from build123d import *

# Parameters (mm, degrees)
SKETCH1_W               = 50
SKETCH1_H               = 100
BOSS_EXTRUDE1_DEPTH     = 10
CUT_EXTRUDE1_DEPTH      = 72.414284285
CUT_EXTRUDE1_DEPTH_BACK = 72.414284285
SKETCH2_R               = 3.104362215
SKETCH2_R_2             = 3.085158395
SKETCH2_R_3             = 3.1
SKETCH2_R_4             = 3.004524649
CUT_EXTRUDE2_DEPTH      = 72.414284285
CUT_EXTRUDE2_DEPTH_BACK = 72.414284285
SKETCH4_R               = 1.557412487
SKETCH4_R_2             = 1.55


with BuildPart() as part:
    # Sketch1 → Boss-Extrude1 (new body)
    with BuildSketch(Plane(origin=(0, 0, 0), x_dir=(1, 0, 0), z_dir=(0, 1, 0))):
        with Locations((-25, 0)):
            Rectangle(SKETCH1_W, SKETCH1_H)
    extrude(amount=BOSS_EXTRUDE1_DEPTH)

    # Sketch2 → Cut-Extrude1 (cut, two sides: drawn at the far end of the back side and taken through both)
    with BuildSketch(Plane(origin=(0, 10, 0), x_dir=(1, 0, 0), z_dir=(0, 1, 0)).offset(-CUT_EXTRUDE1_DEPTH_BACK)):
        with Locations(Location((-32.847308623, -43.305370298, 0), (0, 0, 270))):
            Circle(SKETCH2_R)
        with Locations(Location((-43.698787397, -32.453891525, 0), (0, 0, 270))):
            Circle(SKETCH2_R_2)
        with Locations(Location((-21.99582985, -32.453891525, 0), (0, 0, 270))):
            Circle(SKETCH2_R_3)
        with Locations(Location((-32.847308623, -21.602412752, 0), (0, 0, 270))):
            Circle(SKETCH2_R)
        with Locations(Location((-32.847308623, -32.453891525, 0), (0, 0, 270))):
            Circle(SKETCH2_R_4)
        with Locations(Location((-32.847308623, 32.453891525, 0), (0, 0, 270))):
            Circle(SKETCH2_R_4)
        with Locations(Location((-32.847308623, 21.602412752, 0), (0, 0, 270))):
            Circle(SKETCH2_R)
        with Locations(Location((-21.99582985, 32.453891525, 0), (0, 0, 270))):
            Circle(SKETCH2_R_3)
        with Locations(Location((-43.698787397, 32.453891525, 0), (0, 0, 270))):
            Circle(SKETCH2_R_2)
        with Locations(Location((-32.847308623, 43.305370298, 0), (0, 0, 270))):
            Circle(SKETCH2_R)
    extrude(amount=CUT_EXTRUDE1_DEPTH + CUT_EXTRUDE1_DEPTH_BACK, mode=Mode.SUBTRACT)

    # Sketch4 → Cut-Extrude2 (cut, two sides: drawn at the far end of the back side and taken through both)
    with BuildSketch(Plane(origin=(0, 10, 0), x_dir=(1, 0, 0), z_dir=(0, 1, 0)).offset(-CUT_EXTRUDE2_DEPTH_BACK)):
        with Locations(Location((-41.474384237, 10.515205344, 0), (0, 0, 270))):
            Circle(SKETCH4_R)
        with Locations(Location((-41.474384237, -10.343457517, 0), (0, 0, 270))):
            Circle(SKETCH4_R_2)
        with Locations(Location((-31.474384237, -10.343457517, 0), (0, 0, 270))):
            Circle(SKETCH4_R_2)
        with Locations(Location((-31.474384237, 10.515205344, 0), (0, 0, 270))):
            Circle(SKETCH4_R)
        with Locations(Location((-21.474384237, 10.515205344, 0), (0, 0, 270))):
            Circle(SKETCH4_R_2)
        with Locations(Location((-21.474384237, -10.343457517, 0), (0, 0, 270))):
            Circle(SKETCH4_R_2)
        with Locations(Location((-11.474384237, -10.343457517, 0), (0, 0, 270))):
            Circle(SKETCH4_R_2)
        with Locations((-1.474384237, -10.343457517)):
            Circle(SKETCH4_R_2)
        with Locations(Location((-11.474384237, 10.515205344, 0), (0, 0, 270))):
            Circle(SKETCH4_R)
        with Locations((-1.474384237, 10.515205344)):
            Circle(SKETCH4_R)
    extrude(amount=CUT_EXTRUDE2_DEPTH + CUT_EXTRUDE2_DEPTH_BACK, mode=Mode.SUBTRACT)


solid = part.part
Verification items for the finished model (mm, model axes). Coordinates: 2 decimals unless noted, no trailing zeros. Loops run counter-clockwise (first coordinate to the right, second up) from the corner with the lowest first, then second, coordinate; pieces in that order, holes last. Notation, with made-up numbers: (82.25, 53.25) -> (110.25, 53.25) arc R33 ccw to (110.25, 84.25) -> close; hole circle Ø5 at (37.5, -13). An arc over 180 degrees is marked (long way). Answer as CSV lines item,"result".
1) Cross-section at C-C, the plane y = 6. Count the separate pieces of the cut face and the enclosed holes in it, then the cut area to 3 significant figures.
Found:
separate pieces,"1"
enclosed holes,"18"
area,"4,630 mm2"
2) Release check for a two-part mould opening along Z. For faces 1 (the flat face through (-25, 0, -1)), 2 (the flat face through (-25, 5, -50)), 3 (the cylindrical face through (-35.78, 4.93, 31.8)), 4 (the flat face through (-25, 5, 50)) record: +Z half, -Z half, draft (parallel to the pull), parting line (faces both ways), or undercut.
Found:
face 1,"draft"
face 2,"-Z half"
face 3,"undercut"
face 4,"+Z half"
3) Cross-section at A-A, the plane z = -33.5. Record the cut outline in (x, y).
Found:
outline,"(-50, 0) -> (-46.6, 0) -> (-46.6, 10) -> (-50, 10) -> close; (-40.8, 0) -> (-35.66, 0) -> (-35.66, 10) -> (-40.8, 10) -> close; (-30.03, 0) -> (-24.91, 0) -> (-24.91, 10) -> (-30.03, 10) -> close; (-19.08, 0) -> (0, 0) -> (0, 10) -> (-19.08, 10) -> close"
4) Cross-section at B-B, the plane z = -21. Record the cut outline in (x, y), then the cut area to 3 significant figures.
Found:
outline,"(-50, 0) -> (-35.89, 0) -> (-35.89, 10) -> (-50, 10) -> close; (-29.8, 0) -> (0, 0) -> (0, 10) -> (-29.8, 10) -> close"
area,"439 mm2"
5) Thickness scan on L1, parallel to Z at x = -46.5, y = 6.5; L2, parallel to Z at x = -41, y = 3.25; L3, parallel to X at y = 7.25, z = 30.5. Record the ranges inside material, lowest first. Write a range as from..to.
Found:
L1,"z = -50..-33.75, -31.16..31.16, 33.75..50"
L2,"z = -50..-33.95, -30.96..-12, -9.03..8.87, 11.82..30.96, 33.95..50"
L3,"x = -50..-46.09, -41.31..-35.13, -30.56..-24.4, -19.59..0"
